from build123d import *

# Parameters (mm, degrees)
SKETCH1_R            = 2.5
BOSS_EXTRUDE1_DEPTH  = 10
SKETCH2_R            = 9
MOTORMOUNTBORE_DEPTH = 87.168439698


with BuildPart() as part:
    # Sketch1 → Boss-Extrude1 (new body)
    with BuildSketch(Plane(origin=(0, 0, 0), x_dir=(1, 0, 0), z_dir=(0, 1, 0))):
        with BuildLine():
            Line((-10, -75), (-10, 75))
            ThreePointArc((-10, 75), (0, 85), (10, 75))
            Line((10, 75), (10, -75))
            ThreePointArc((10, -75), (0, -85), (-10, -75))
        make_face()
        with Locations(Location((0, 75, 0), (0, 0, 270))):
            Circle(SKETCH1_R, mode=Mode.SUBTRACT)
        with Locations(Location((0, -75, 0), (0, 0, 270))):
            Circle(SKETCH1_R, mode=Mode.SUBTRACT)
    extrude(amount=BOSS_EXTRUDE1_DEPTH)

    # Sketch2 → MotorMountBore (cut, through all)
    with BuildSketch(Plane(origin=(0, 10, 0), x_dir=(1, 0, 0), z_dir=(0, 1, 0))):
        with Locations(Location((0, 25, 0), (0, 0, 270))):
            Circle(SKETCH2_R)
    extrude(amount=-MOTORMOUNTBORE_DEPTH, mode=Mode.SUBTRACT)


solid = part.part
Can you work these out from the model? Positions are in its coordinate system, mm. Round coordinates to 2 decimals unless told otherwise and drop trailing zeros. Order: outer loops, then holes, each group sorted by start corner. A loop starts at its lowest first (then second) coordinate and runs counter-clockwise, first axis right, second up. Notation, with made-up numbers: (32.5, 30.5) -> (59.5, 30.5) arc R19 cw to (59.5, 67.5) -> close; hole circle Ø3 at (52, 81). An arc over 180 degrees is marked (long way). Write each question's results on one line, items separated by ' | '. Start each with the question number.
Item 1: If we section it at B-B, the plane x = 0: Write out the boundary of the cut face in (y, z).
Item 2: Please list where these lines run through material, in increasing order: L1, parallel to X at y = 7, z = -75; L2, parallel to X at y = 3.5, z = -25; L3, parallel to Z at x = 0.75, y = 2.25.
Item 3: Will these pins go through, and if not, where does the flat tip stop? pin 1 (2 mm diameter, centred on x = -3.5, y = 3, fed in from -Z); pin 2 (4 mm diameter, centred on x = 7, y = 2.5, fed in from -Z).
Item 4: If we section it at C-C, the plane y = 7: Write out the boundary of the cut face in (x, z).
Item 5: If we section it at A-A, the plane z = -25: Write out the boundary of the cut face in (x, y).
Item 6: Thinking about a two-plate mould opening in Z: for faces 1 (the cylindrical face through (0.1, 4.9, -77.5)), 2 (the cylindrical face through (0, 5, -85)), 3 (the flat face through (-10, 5, 1)), 4 (the cylindrical face through (0, 5, 85)), which applies, +Z half, -Z half, draft (parallel to the pull), parting line (faces both ways), or undercut?
Results:
1) outline: (0, -85) -> (10, -85) -> (10, -77.5) -> (0, -77.5) -> close; (0, -72.5) -> (10, -72.5) -> (10, -34) -> (0, -34) -> close; (0, -16) -> (10, -16) -> (10, 72.5) -> (0, 72.5) -> close; (0, 77.5) -> (10, 77.5) -> (10, 85) -> (0, 85) -> close
2) L1: x = -10 to -2.5, 2.5 to 10 | L2: x = -10 to -9, 9 to 10 | L3: z = -84.97 to -77.38, -72.62 to -33.97, -16.03 to 72.62, 77.38 to 84.97
3) pin 1: stops at z = -84.68 | pin 2: stops at z = -83.66
4) outline: (-10, -75) arc R10 ccw to (10, -75) -> (10, 75) arc R10 ccw to (-10, 75) -> close; hole circle Ø18 at (0, -25); hole circle Ø5 at (0, -75); hole circle Ø5 at (0, 75)
5) outline: (-10, 0) -> (-9, 0) -> (-9, 10) -> (-10, 10) -> close; (9, 0) -> (10, 0) -> (10, 10) -> (9, 10) -> close
6) face 1: undercut | face 2: -Z half | face 3: draft | face 4: +Z half
